from build123d import *

# Parameters (mm, degrees)
SKETCH1_R               = 3.175
BOSS_EXTRUDE1_DEPTH     = 18.415
SKETCH2_R               = 1.4478
BOSS_EXTRUDE2_DEPTH     = 5.3975
FILLET1_R               = 1.5875
CUT_EXTRUDE1_DEPTH      = 25.232135817
CUT_EXTRUDE1_DEPTH_BACK = 25.232135817
SKETCH3_R               = 1.397


with BuildPart() as part:
    # Sketch1 → Boss-Extrude1 (new body)
    with BuildSketch(Plane.XY):
        Circle(SKETCH1_R)
    extrude(amount=BOSS_EXTRUDE1_DEPTH)

    # Sketch2 → Boss-Extrude2 (add)
    with BuildSketch(Plane.XY.offset(18.415)):
        Circle(SKETCH2_R)
    extrude(amount=BOSS_EXTRUDE2_DEPTH)

    # Fillet1
    fillet1_edges = [part.edges().sort_by_distance(p)[0] for p in [
        (-1.4478, 0, 18.415),
    ]]
    fillet(fillet1_edges, radius=FILLET1_R)

    # Sketch3 → Cut-Extrude1 (cut, two sides: drawn at the far end of the back side and taken through both)
    with BuildSketch(Plane(origin=(0, 0, 0), x_dir=(1, 0, 0), z_dir=(0, 1, 0)).offset(-CUT_EXTRUDE1_DEPTH_BACK)):
        with Locations(Location((0, -3.175, 0), (0, 0, 270))):
            Circle(SKETCH3_R)
    extrude(amount=CUT_EXTRUDE1_DEPTH + CUT_EXTRUDE1_DEPTH_BACK, mode=Mode.SUBTRACT)


solid = part.part
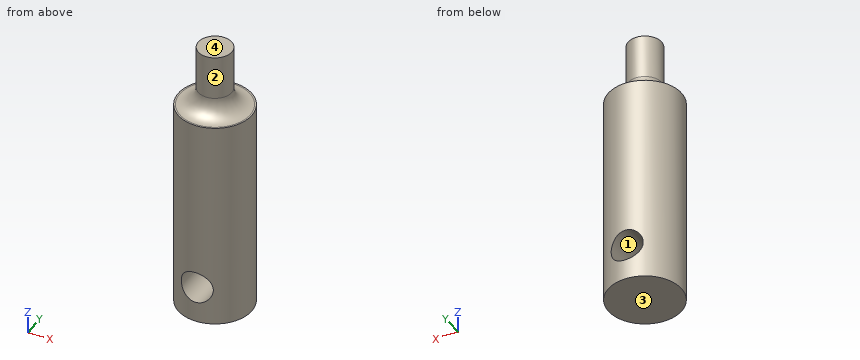
Here's how the part is built. I have some questions about the finished solid (model axes, mm). Face numbers are marked on the shaded views. Give positions to 0.01 mm unless a question says otherwise; leave off trailing zeros. Loops run counter-clockwise (first coordinate to the right, second up) from the corner with the lowest first, then second, coordinate; pieces in that order, holes last. Notation, with made-up numbers: (64.5, 6) -> (68.5, 6) arc R27 ccw to (68.5, 35) -> close; hole circle Ø11 at (-17.5, 62). An arc over 180 degrees is marked (long way). Answer as a JSON object with one key per item and string values. Group by question number.
Item 1: Thinking about a two-plate mould opening in Z: for the marked faces 1, 2, 3 and 4, which applies, pulls with the +Z half, pulls with the -Z half, needs draft (parallel to the pull), parting line crosses it, or undercut?
Item 2: I need wall thicknesses on L1, parallel to Z at x = 0, y = -1.75; L2, parallel to Z at x = 0.5, y = -2.5; L3, parallel to X at y = 2.75, z = 4. Which ranges of each line are inside material? Lowest first, please.
Item 3: Imagine slicing it at C-C on z = 10.75. Write out the boundary of the cut face in (x, y) (3 decimals), then the cut area to 3 significant figures.
Item 4: Will these pins go through, and if not, where does the flat tip stop? pin 1 (1 mm diameter, centred on x = 1.5, y = -2, fed in from +Z); pin 2 (1 mm diameter, centred on x = -2, z = 2.5, fed in from -Y).
Answer list:
{
 "1": {"face 1": "undercut", "face 2": "needs draft", "face 3": "pulls with the -Z half", "face 4": "pulls with the +Z half"},
 "2": {"L1": "z = 0 to 1.78, 4.57 to 19.07", "L2": "z = 0 to 1.87, 4.48 to 18.49", "L3": "x = -1.59 to -1.13, 1.13 to 1.59"},
 "3": {"outline": "circle Ø6.35 at (0, 0)", "area": "31.7 mm2"},
 "4": {"pin 1": "stops at z = 18.8", "pin 2": "stops at y = -2.8"}
}
